CAD build for the part. Positions are in the model's coordinates, mm. Face numbers are marked on the shaded views. Give positions to 0.01 mm unless a question says otherwise; leave off trailing zeros. Order: outer loops, then holes, each group sorted by start corner. A loop starts at its lowest first (then second) coordinate and runs counter-clockwise, first axis right, second up. Notation, with made-up numbers: (42, 22.5) -> (46, 22.5) arc R21 ccw to (46, 59.5) -> close; hole circle Ø11 at (-29, 53.25). An arc over 180 degrees is marked (long way). Use one line per item in the form item = value. Start each with the question number.
1) Mould opens along Y. For the marked faces 1, 2, 3 and 4 say: pulls with the +Y half, pulls with the -Y half, needs draft (parallel to the pull), parting line crosses it, or undercut.
2) Cut at B-B, the plane y = 919. Give the cut face in (x, z).
3) Drop flat-ended pins along their axis: P1, Ø1.5, axis at y = 287, z = 57.5, coming from the -X side; P2, Ø6, axis at x = 94, y = 474.5, coming from the -Z side; P3, Ø10, axis at x = 129, z = 108.5, coming from the +Y side; P4, Ø1.5, axis at x = 37, y = 509.5, coming from the +Z side. Give the stop position or say it passes through.
4) Cut at A-A, the plane z = -504.5. Give the cut face in (x, y).
5) Probe line 1 (Y direction, x = 121, z = 42.5); line 2 (Z direction, x = 141.5, y = -515); line 3 (Z direction, x = 31.5, y = -761). List the from-to ranges inside material, lowest first.
6) Cut at C-C, the plane x = 58. State how many separate pieces and enclosed holes the cut face has, and give its area (3 significant figures).
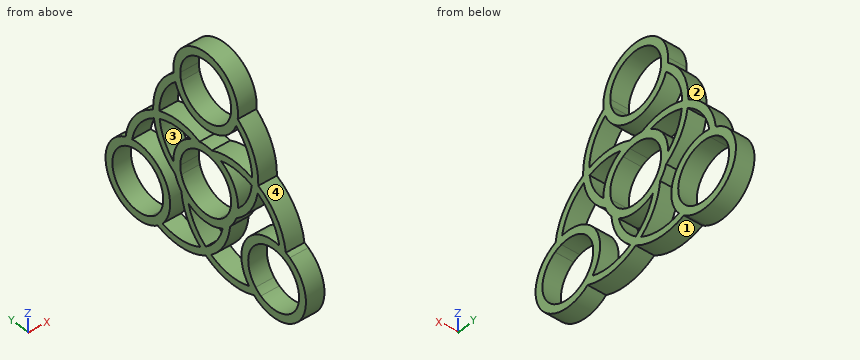
from build123d import *

# Parameters (mm, degrees)
F1_DEPTH = 177.8
F2_COUNT = 3


with BuildPart() as f1:
    # F0 (on Right) → F1 (new body)
    with BuildSketch(Plane.YZ):
        with BuildLine():
            ThreePointArc((-268.4926933874, -79.5693082951), (-313.7669030634, -48.1461873832), (-355.396348822, -12.0330895451))
            ThreePointArc((-355.396348822, -12.0330895451), (-349.6172674569, -64.9548019471), (-336.0023494952, -116.4207074952))
            ThreePointArc((-336.0023494952, -116.4207074952), (-275.6466077337, -154.0273882117), (-211.1384628897, -183.9569262452))
            ThreePointArc((-211.1384628897, -183.9569262452), (-245.4296339346, -134.8476770721), (-268.4926933874, -79.5693082951))
        make_face()
        with BuildLine():
            ThreePointArc((-336.0023494952, -116.4207074952), (-349.6172674569, -64.9548019471), (-355.396348822, -12.0330895451))
            ThreePointArc((-355.396348822, -12.0330895451), (-511.134133308, 369.8320431433), (-334.3887781327, 742.4394994612))
            ThreePointArc((-334.3887781327, 742.4394994612), (-345.3149861043, 778.5114296956), (-352.361893863, 815.5371945428))
            ThreePointArc((-352.361893863, 815.5371945428), (-579.3079627247, 345.4308557736), (-336.0023494952, -116.4207074952))
        make_face()
        with BuildLine():
            ThreePointArc((511.3322337625, 355.6), (470.7367959904, 155.9314692167), (355.396348822, -12.0330895451))
            ThreePointArc((355.396348822, -12.0330895451), (349.6172674569, -64.9548019471), (336.0023494952, -116.4207074952))
            ThreePointArc((336.0023494952, -116.4207074952), (514.9659945491, 90.0606401517), (579.3972101854, 355.6))
            ThreePointArc((579.3972101854, 355.6), (519.5472189563, 612.0601615171), (352.361893863, 815.5371945428))
            ThreePointArc((352.361893863, 815.5371945428), (345.3149861043, 778.5114296956), (334.3887781327, 742.4394994612))
            ThreePointArc((334.3887781327, 742.4394994612), (464.9969968463, 568.2933149123), (511.3322337625, 355.6))
        make_face()
        with BuildLine():
            ThreePointArc((336.0023494952, -116.4207074952), (349.6172674569, -64.9548019471), (355.396348822, -12.0330895451))
            ThreePointArc((355.396348822, -12.0330895451), (313.7669030634, -48.1461873832), (268.4926933874, -79.5693082951))
            ThreePointArc((268.4926933874, -79.5693082951), (245.4296339346, -134.8476770721), (211.1384628897, -183.9569262452))
            ThreePointArc((211.1384628897, -183.9569262452), (275.6466077337, -154.0273882117), (336.0023494952, -116.4207074952))
        make_face()
        with BuildLine():
            ThreePointArc((-211.1384628897, -183.9569262452), (-275.6466077337, -154.0273882117), (-336.0023494952, -116.4207074952))
            ThreePointArc((-336.0023494952, -116.4207074952), (0, -355.6), (336.0023494952, -116.4207074952))
            ThreePointArc((336.0023494952, -116.4207074952), (275.6466077337, -154.0273882117), (211.1384628897, -183.9569262452))
            ThreePointArc((211.1384628897, -183.9569262452), (0, -280.035), (-211.1384628897, -183.9569262452))
        make_face()
        with BuildLine():
            ThreePointArc((-352.361893863, 815.5371945428), (-345.3149861043, 778.5114296956), (-334.3887781327, 742.4394994612))
            ThreePointArc((-334.3887781327, 742.4394994612), (-303.2012975673, 767.3397557172), (-270.1668730977, 789.7319084854))
            ThreePointArc((-270.1668730977, 789.7319084854), (-277.5178808464, 825.9544493975), (-280.0343843816, 862.8296035669))
            ThreePointArc((-280.0343843816, 862.8296035669), (-317.0810719236, 840.5337284603), (-352.361893863, 815.5371945428))
        make_face()
        with BuildLine():
            ThreePointArc((355.6, 863.4167909622), (-23.994484182, 1218.2063408771), (-352.361893863, 815.5371945428))
            ThreePointArc((-352.361893863, 815.5371945428), (-317.0810719236, 840.5337284603), (-280.0343843816, 862.8296035669))
            ThreePointArc((-280.0343843816, 862.8296035669), (-0.293593859, 1143.4516370576), (280.035, 863.4167909622))
            ThreePointArc((280.035, 863.4167909622), (280.0348460953, 863.1231971032), (280.0343843816, 862.8296035669))
            ThreePointArc((280.0343843816, 862.8296035669), (317.0810719236, 840.5337284603), (352.361893863, 815.5371945428))
            ThreePointArc((352.361893863, 815.5371945428), (354.7895499149, 839.4223067802), (355.6, 863.4167909622))
        make_face()
        with BuildLine():
            ThreePointArc((270.1668730977, 789.7319084854), (303.2012975673, 767.3397557172), (334.3887781327, 742.4394994612))
            ThreePointArc((334.3887781327, 742.4394994612), (345.3149861043, 778.5114296956), (352.361893863, 815.5371945428))
            ThreePointArc((352.361893863, 815.5371945428), (317.0810719236, 840.5337284603), (280.0343843816, 862.8296035669))
            ThreePointArc((280.0343843816, 862.8296035669), (277.5178808464, 825.9544493975), (270.1668730977, 789.7319084854))
        make_face()
        with BuildLine():
            ThreePointArc((-270.1668730977, 789.7319084854), (-303.2012975673, 767.3397557172), (-334.3887781327, 742.4394994612))
            ThreePointArc((-334.3887781327, 742.4394994612), (0, 507.8167909622), (334.3887781327, 742.4394994612))
            ThreePointArc((334.3887781327, 742.4394994612), (303.2012975673, 767.3397557172), (270.1668730977, 789.7319084854))
            ThreePointArc((270.1668730977, 789.7319084854), (0, 583.3817909622), (-270.1668730977, 789.7319084854))
        make_face()
        with BuildLine():
            ThreePointArc((355.396348822, -12.0330895451), (355.5490835603, -6.0174063724), (355.6, 0))
            ThreePointArc((355.6, 0), (-6.0174063724, 355.5490835603), (-355.396348822, -12.0330895451))
            ThreePointArc((-355.396348822, -12.0330895451), (-313.7669030634, -48.1461873832), (-268.4926933874, -79.5693082951))
            ThreePointArc((-268.4926933874, -79.5693082951), (-40.2010561568, 277.1344011646), (280.035, 0))
            ThreePointArc((280.035, 0), (277.1344011646, -40.2010561568), (268.4926933874, -79.5693082951))
            ThreePointArc((268.4926933874, -79.5693082951), (313.7669030634, -48.1461873832), (355.396348822, -12.0330895451))
        make_face()
    extrude(amount=F1_DEPTH)

    # F2: F1 ×3 about axis
    f2_axis = Axis((0, -4e-10, 0), (-1, 0, 0))


with BuildPart() as f1_1:
    add(f1.part)
    for i in range(1, F2_COUNT):
        add(f1.part.rotate(f2_axis, i * 360 / F2_COUNT))


solid = f1_1.part
Result:
q1.face_1 = undercut
q1.face_2 = pulls with the +Y half
q1.face_3 = undercut
q1.face_4 = pulls with the -Y half
q2.outline = (0, -743.35) -> (177.8, -743.35) -> (177.8, -653.27) -> (0, -653.27) -> close; (0, -210.15) -> (177.8, -210.15) -> (177.8, -120.06) -> (0, -120.06) -> close
q3.P1 = 0
q3.P2 = -733.64
q3.P3 = 814.49
q3.P4 = 632.86
q4.outline = (0, -1095.81) -> (177.8, -1095.81) -> (177.8, -1018.15) -> (0, -1018.15) -> close; (0, -477.33) -> (177.8, -477.33) -> (177.8, -399.67) -> (0, -399.67) -> close; (0, -170.55) -> (177.8, -170.55) -> (177.8, -85.4) -> (0, -85.4) -> close; (0, 85.4) -> (177.8, 85.4) -> (177.8, 170.55) -> (0, 170.55) -> close; (0, 399.67) -> (177.8, 399.67) -> (177.8, 477.33) -> (0, 477.33) -> close; (0, 1018.15) -> (177.8, 1018.15) -> (177.8, 1095.81) -> (0, 1095.81) -> close
q5.line_1 = -843.84 to -769.4, -487.51 to -404.26, -353.05 to -276.79, 276.79 to 353.05, 404.26 to 487.51, 769.4 to 843.84
q5.line_2 = -718.94 to -587.44, -275.98 to -162.85, 90.13 to 621.07
q5.line_3 = -787.06 to -711.43, -151.99 to -76.36, 59.3 to 183.39
q6.separate_pieces = 1
q6.enclosed_holes = 10
q6.area = 981,000 mm²
